Geometry: final body of the model. Coordinates: model frame, mm. Face numbers are marked on the shaded views. A direction names the side the tool comes from. Give positions to 0.01 mm unless a question says otherwise; leave off trailing zeros. Write each loop counter-clockwise with the first axis right and the second up, starting at its lowest first coordinate (ties: lowest second). Pieces come first, ordered by that corner, then holes.
Q1. Pin query (flat end, axial travel): pin 1 (4 mm diameter, centred on x = -15.5, z = 19.5, fed in from +Y); pin 2 (6 mm diameter, centred on x = 9.5, z = 26.5, fed in from +Y); pin 3 (6 mm diameter, centred on x = -18, y = -26.5, fed in from +Z). Return the tip coordinate at first contact, or that it passes through.
Q2. Cut plane A-A on z = 19.9. Count the separate pieces of the cut face and the enclosed holes in it, plus the area to 3 significant figures.
Q3. Cut plane D-D on y = 20. Return the cut outline in (x, z), plus the area to 3 significant figures.
Q4. Draft query along X for the marked faces 1, 2, 3 and 4. Return one class per face: pulls with the +X half, pulls with the -X half, needs draft (parallel to the pull), parting line crosses it, or undercut.
Q5. Cut plane B-B on y = -15.5. Return the cut outline in (x, z), plus the area to 3 significant figures.
Q6. Cut plane C-C on x = 6.5. Return the cut outline in (y, z).
Q7. Line query: L1, parallel to X at y = -25, z = 20.5; L2, parallel to X at y = -28.7, z = 19.9; L3, parallel to Y at x = -44.5, z = 19.9. Output: solid intervals per line, ascending.
Q8. Reachability of the marked faces 5, 6 and 7 from +Z, -Z, +X, -X, +Y, -Y: full face, straight path, thin tool, end or side. Return the list, or none.
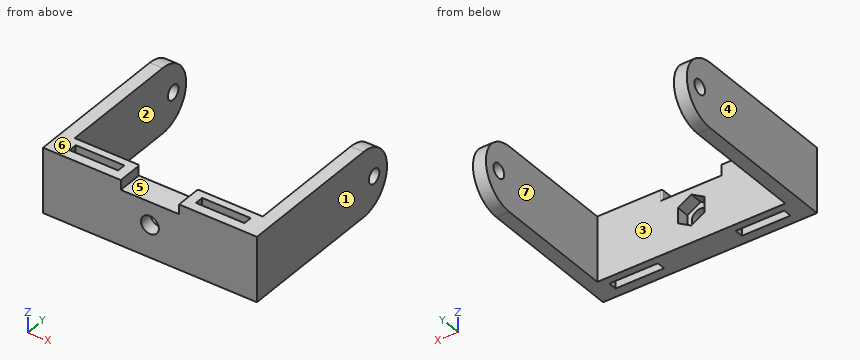
```python
from build123d import *

# Parameters (mm, degrees)
SKETCH005_W             = 58
SKETCH005_H             = 20
SKETCH005_R             = 2.75
PAD004_DEPTH            = 8
SKETCH006_R             = 2.25
PAD005_DEPTH            = 4
POCKET005_DEPTH         = 4
SKETCH011_W             = 15
SKETCH011_H             = 2.666667
POCKET007_DEPTH         = 20
SKETCH012_W             = 18
SKETCH012_H             = 3
POCKET008_DEPTH         = 8
FILLET_R                = 0.5
BODY002_PLACEMENT_ANGLE = 180


with BuildPart() as part:
    # Sketch005 → Pad004 (new body)
    with BuildSketch(Plane.XZ):
        Rectangle(SKETCH005_W, SKETCH005_H)
        Circle(SKETCH005_R, mode=Mode.SUBTRACT)
    extrude(amount=PAD004_DEPTH)

    # Sketch006 (on Face4 of Pad004) → Pad005 (join)
    with BuildSketch(Plane(origin=(-29, 0, 0), x_dir=(0, 0, -1), z_dir=(-1, 0, 0))):
        with BuildLine():
            Line((-10, 0), (10, 0))
            Line((10, 0), (10, 45.5))
            ThreePointArc((10, 45.5), (0, 55.5), (-10, 45.5))
            Line((-10, 45.5), (-10, 0))
        make_face()
        with Locations((0, 50)):
            Circle(SKETCH006_R, mode=Mode.SUBTRACT)
    pad005 = extrude(amount=PAD005_DEPTH)

    # Mirrored003: Pad005 across YZ
    add(pad005.mirror(Plane.YZ))

    # Sketch007 (on Face5 of Mirrored003) → Pocket005 (cut)
    with BuildSketch(Plane.XZ.offset(8)):
        Polygon((4.113621, 2.375), (0, 4.75), (-4.113621, 2.375), (-4.113621, -2.375), (0, -4.75), (4.113621, -2.375), align=None)
    extrude(amount=-POCKET005_DEPTH, mode=Mode.SUBTRACT)

    # Sketch011 (on Face14 of Pocket005) → Pocket007 (cut)
    with BuildSketch(Plane(origin=(0, 0, 10), x_dir=(-1, 0, 0), z_dir=(0, 0, 1))):
        with Locations((-19.5, 4.333334)):
            Rectangle(SKETCH011_W, SKETCH011_H)
    pocket007 = extrude(amount=-POCKET007_DEPTH, mode=Mode.SUBTRACT)

    # Mirrored004: Pocket007 across YZ
    add(pocket007.mirror(Plane.YZ), mode=Mode.SUBTRACT)

    # Sketch012 (on Face3 of Mirrored004) → Pocket008 (cut)
    with BuildSketch(Plane(origin=(0, 0, 0), x_dir=(1, 0, 0), z_dir=(0, 1, 0))):
        with Locations((0, 8.5)):
            Rectangle(SKETCH012_W, SKETCH012_H)
    extrude(amount=-POCKET008_DEPTH, mode=Mode.SUBTRACT)

    # Fillet
    fillet_edges = [part.edges().sort_by_distance(p)[0] for p in [
        (0, -8, -7),
        (9, -8, -8.5),
        (-9, -8, -8.5),
    ]]
    fillet(fillet_edges, radius=FILLET_R)


with BuildPart() as part_1:
    # Body002 placement: moved
    add(part.part.moved(Location((-14.3, -30, 19.9))).rotate(Axis((-14.3, -30, 19.9), (1, 0, 0)), BODY002_PLACEMENT_ANGLE))


solid = part_1.part
```
Data:
1. pin 1: stops at y = -26
1. pin 2: stops at y = -22
1. pin 3: stops at z = 26.9
2. separate pieces: 4
2. enclosed holes: 2
2. area: 737 mm2
3. outline: (-47.3, 10.97) - (-43.3, 10.97) - (-43.3, 17.65) - (-47.3, 17.65) - close; (-47.3, 22.15) - (-43.3, 22.15) - (-43.3, 28.83) - (-47.3, 28.83) - close; (14.7, 10.97) - (18.7, 10.97) - (18.7, 17.65) - (14.7, 17.65) - close; (14.7, 22.15) - (18.7, 22.15) - (18.7, 28.83) - (14.7, 28.83) - close
3. area: 107 mm2
4. face 1: pulls with the +X half
4. face 2: undercut
4. face 3: undercut
4. face 4: pulls with the -X half
5. outline: (-47.3, 9.9) - (-43.3, 9.9) - (-43.3, 29.9) - (-47.3, 29.9) - close; (14.7, 9.9) - (18.7, 9.9) - (18.7, 29.9) - (14.7, 29.9) - close
5. area: 160 mm2
6. outline: (-30, 9.9) - (-27, 9.9) - (-27, 29.9) - (-30, 29.9) - close; (-24.33, 9.9) - (-22, 9.9) - (-22, 29.9) - (-24.33, 29.9) - close
7. L1: x = -47.3 to -41.3, -26.3 to -18.41, -10.19 to -2.3, 12.7 to 18.7
7. L2: x = -47.3 to -17.05, -11.55 to 18.7
7. L3: y = -30 to 17.75, 22.25 to 25.5
8. face 5: +Z, +Y, -Y
8. face 6: +Z, +X, -X, +Y, -Y
8. face 7: +Z, -Z, +Y
